Check sheet for the modelled part. Datum: model origin and axes. Units: mm. A direction names the side the tool comes from. Round coordinates to 2 decimals unless told otherwise and drop trailing zeros. Write each loop counter-clockwise with the first axis right and the second up, starting at its lowest first coordinate (ties: lowest second). Pieces come first, ordered by that corner, then holes.
Item 1: Cross-section at C-C on z = 0.65. Count the separate pieces of the cut face and the enclosed holes in it, plus the area to 3 significant figures.
Item 2: Release check for a two-part mould opening along Y. For faces 3 (the cylindrical face through (-38.72, 57.27, 0.99)), 4 (the cylindrical face through (41.02, 53.406, 1.014)), 5 (the cylindrical face through (31.9, 2.4, 1)) record: +Y half, -Y half, draft (parallel to the pull), parting line (faces both ways), or undercut.
Item 3: Cross-section at A-A on x = -12. Enter the section's corners in (y, z).
Item 4: Cross-section at B-B on y = 9. Enter the section's corners in (x, z), plus the area to 3 significant figures.
Item 5: Material ranges on line 1 (X direction, y = 46, z = 1.5); line 2 (X direction, y = 39.5, z = 1.3); line 3 (Y direction, x = 6.5, z = 1.3), recorded low to high.
Item 6: Cross-section at D-D on y = 65.5. Enter the section's corners in (x, z), plus the area to 3 significant figures.
Item 7: Tool access check on faces 1 (the flat face through (7.21, 73.23, 1.01)), 2 (the cylindrical face through (46.193, 31.142, 0.986)). Record the directions out of +Z, -Z, +X, -X, +Y, -Y that give a thin tool (end or side, any length) a straight path to the whole face; none if there is none.
Item 8: Go/stop test with flat-tipped pins: pin 1 Ø1 at (x, z) = (18.5, 0) entering from -Y; pin 2 Ø1 at (x, z) = (15, 1.5) entering from +Y. Record where each tip stops, or that it passes through.
Autodesk Inventor part; units mm, degrees
ref_plane "YZ Plane" through (0, 0, 0) normal (1, 0, 0) x (0, 1, 0)
ref_plane "XZ Plane" through (0, 0, 0) normal (0, 1, 0) x (-1, 0, 0)
ref_plane "XY Plane" through (0, 0, 0) normal (0, 0, 1) x (1, 0, 0)
ref_plane "Arbeitsebene1" through (0, 0, 0) normal (0, 0, 1) x (1, 0, 0)
sketch "Skizze1" plane through (0, 0, 0) normal (0, 0, 1) x (1, 0, 0)
  line L0 (39.3233, 58.7442) -> (31.1975, 48.5587)
  arc A0 (20.3661, 6.7006) -> (31.1975, 48.5587) centre (0, 34.301) ccw
  line L1 (20.3661, 6.7006) -> (24.3422, 1.3125)
  arc A1 (24.3422, 1.3125) -> (31.7994, 0.6471) centre (28.3654, 4.2814) ccw
  arc A2 (31.7994, 0.6471) -> (39.3233, 58.7442) centre (0, 34.301) ccw
  circle A3 centre (37.5836, 49.0481) radius 1.4
  circle A4 centre (39.9219, 28.2806) radius 1.4
  circle A5 centre (31.5631, 9.1262) radius 1.4
  line L2 (6.9617, 67.8882) -> (15.0883, 78.0746)
  arc A6 (15.0883, 78.0746) -> (-39.8826, 57.8205) centre (0, 34.301) ccw
  arc A7 (-39.8826, 57.8205) -> (-37.5755, 50.698) centre (-35.5757, 55.2807) ccw
  line L3 (-37.5755, 50.698) -> (-31.4381, 48.0198)
  arc A8 (6.9617, 67.8882) -> (-31.4381, 48.0198) centre (0, 34.301) ccw
  circle A9 centre (-31.5631, 59.4759) radius 1.4
  circle A10 centre (-14.7471, 71.8847) radius 1.4
  circle A11 centre (6.0205, 74.2229) radius 1.4
  circle A12 centre (-0.002, 34.3021) radius 3.35
  circle A13 centre (9.062, 45.6666) radius 3
  circle A14 centre (2.4174, 50.9675) radius 1.9
  circle A15 centre (15.7065, 40.3657) radius 1.9
  circle A16 centre (6.6446, 29.0001) radius 1.9
  circle A17 centre (-6.6446, 39.602) radius 1.9
  line L4 (31.7994, 0.6471) -> (-40.3324, 56.8214)
  arc A18 (20.3661, 6.7006) -> (-31.4381, 48.0198) centre (0, 34.301) ccw
  arc A19 (31.7994, 0.6471) -> (-39.8826, 57.8205) centre (0, 34.301) ccw
  circle A20 centre (15.7065, 40.3657) radius 1.4
  circle A21 centre (6.6446, 29.0001) radius 1.4
  circle A22 centre (-6.6446, 39.602) radius 1.4
  circle A23 centre (2.4174, 50.9675) radius 1.4
  point P0 (0, 0)
  dimension "d2" = 2.8
  dimension "d3" = 2.8
  dimension "d4" = 2.8
  dimension "d5" = 2.8
extrude "Extrusion1" add sketch "Skizze1" along normal blind 2 contours A2 L4 A0 L0 | L0 A18 L2 A19 | A0 L4 A8 A18 | L2 A8 L4 A7 A6 | A14 | A15 | A16 | A17
sketch "Skizze2" plane through (0, 0, 2) normal (0, 0, 1) x (1, 0, 0)
  arc A0 (31.7994, 0.6471) -> (-39.8826, 57.8205) centre (0, 34.301) ccw
  arc A1 (-39.8826, 57.8205) -> (-40.3324, 56.8214) centre (-35.5757, 55.2807) ccw
  line L0 (-40.3324, 56.8214) -> (31.7994, 0.6471)
  circle A2 centre (31.5631, 9.1262) radius 1.4
  circle A3 centre (39.9219, 28.2806) radius 1.4
  circle A4 centre (37.5836, 49.0481) radius 1.4
  circle A5 centre (-31.5631, 59.4759) radius 1.4
  circle A6 centre (-14.7471, 71.8847) radius 1.4
  circle A7 centre (6.0205, 74.2229) radius 1.4
  circle A8 centre (9.062, 45.6666) radius 3
  circle A9 centre (-0.002, 34.3021) radius 3.35
  circle A10 centre (15.7065, 40.3657) radius 1.4
  circle A11 centre (2.4174, 50.9675) radius 1.4
  circle A12 centre (-6.6446, 39.602) radius 1.4
  circle A13 centre (6.6446, 29.0001) radius 1.4
  line L1 (29.1054, 5.9703) -> (34.0209, 12.2821) construction
  circle A14 centre (31.5631, 9.1262) radius 1.4
  line L2 (30.3283, 5.018) -> (35.2438, 11.3297)
  line L3 (32.798, 13.2345) -> (27.8825, 6.9227)
  arc A15 (27.8825, 6.9227) -> (30.3283, 5.018) centre (29.1054, 5.9703) ccw
  arc A16 (35.2438, 11.3297) -> (32.798, 13.2345) centre (34.0209, 12.2821) ccw
  line L4 (37.4642, 25.1247) -> (42.3796, 31.4365) construction
  line L5 (38.6871, 24.1723) -> (43.6025, 30.4841)
  line L6 (41.1567, 32.3888) -> (36.2413, 26.0771)
  arc A17 (36.2413, 26.0771) -> (38.6871, 24.1723) centre (37.4642, 25.1247) ccw
  arc A18 (43.6025, 30.4841) -> (41.1567, 32.3888) centre (42.3796, 31.4365) ccw
  line L7 (35.1259, 45.8922) -> (40.0413, 52.204) construction
  line L8 (36.3488, 44.9399) -> (41.2642, 51.2516)
  line L9 (38.8184, 53.1564) -> (33.903, 46.8446)
  arc A19 (33.903, 46.8446) -> (36.3488, 44.9399) centre (35.1259, 45.8922) ccw
  arc A20 (41.2642, 51.2516) -> (38.8184, 53.1564) centre (40.0413, 52.204) ccw
  line L10 (3.5627, 71.0671) -> (8.4782, 77.3788) construction
  line L11 (4.7857, 70.1147) -> (9.7011, 76.4265)
  line L12 (7.2553, 78.3312) -> (2.3398, 72.0194)
  arc A21 (2.3398, 72.0194) -> (4.7857, 70.1147) centre (3.5627, 71.0671) ccw
  arc A22 (9.7011, 76.4265) -> (7.2553, 78.3312) centre (8.4782, 77.3788) ccw
  line L13 (-17.2048, 68.7288) -> (-12.2894, 75.0405) construction
  line L14 (-15.9819, 67.7764) -> (-11.0664, 74.0882)
  line L15 (-13.5123, 75.9929) -> (-18.4277, 69.6811)
  arc A23 (-18.4277, 69.6811) -> (-15.9819, 67.7764) centre (-17.2048, 68.7288) ccw
  arc A24 (-11.0664, 74.0882) -> (-13.5123, 75.9929) centre (-12.2894, 75.0405) ccw
  line L16 (-34.0209, 56.32) -> (-29.1054, 62.6318) construction
  line L17 (-32.798, 55.3676) -> (-27.8825, 61.6794)
  line L18 (-30.3283, 63.5841) -> (-35.2438, 57.2723)
  arc A25 (-35.2438, 57.2723) -> (-32.798, 55.3676) centre (-34.0209, 56.32) ccw
  arc A26 (-27.8825, 61.6794) -> (-30.3283, 63.5841) centre (-29.1054, 62.6318) ccw
  line L19 (29.1054, 5.9703) -> (34.0209, 12.2821) construction
  line L20 (30.3283, 5.018) -> (35.2438, 11.3297)
  line L21 (32.798, 13.2345) -> (27.8825, 6.9227)
  arc A27 (27.8825, 6.9227) -> (30.3283, 5.018) centre (29.1054, 5.9703) ccw
  arc A28 (35.2438, 11.3297) -> (32.798, 13.2345) centre (34.0209, 12.2821) ccw
  point P0 (0, 0)
  dimension "d6" = 4
  dimension "d7" = 3.1
  dimension "d8" = 3.1
  dimension "d9" = 3.1
  dimension "d10" = 3.1
  dimension "d11" = 3.1
  dimension "d12" = 3.1
  dimension "d13" = 3.1
extrude "Extrusion2" cut sketch "Skizze2" against normal blind 2 contours A7 | A15 L3 A16 L2 | A17 L6 A18 L5 | A19 L9 A20 L8 | A21 L12 A22 L11 | A23 L15 A24 L14 | A25 L18 A26 L17
fillet "Rundung1" radius 5 2 edges at (-40.3324, 56.8214, 1) (31.7994, 0.6471, 1)
properties part number "Anglerfish_Lightplate_Tosslink_adjuster_flipped"
Response values:
1. separate pieces: 1
1. enclosed holes: 12
1. area: 3,720 mm2
2. face 3: parting line
2. face 4: undercut
2. face 5: -Y half
3. outline: (34.76, 0) - (72.89, 0) - (72.89, 2) - (34.76, 2) - close; (76.56, 0) - (79.02, 0) - (79.02, 2) - (76.56, 2) - close
4. outline: (21.07, 0) - (29.5, 0) - (29.5, 2) - (21.07, 2) - close; (33.43, 0) - (38.78, 0) - (38.78, 2) - (33.43, 2) - close
4. area: 27.5 mm2
5. line 1: x = -26.44 to 6.08, 12.04 to 33.58, 37.17 to 44.8
5. line 2: x = -18.09 to -8.04, -5.25 to 14.61, 16.81 to 46.01
5. line 3: y = 20.35 to 27.61, 30.39 to 44.11, 47.23 to 72.32, 77.36 to 80.14
6. outline: (-34.21, 0) - (34.21, 0) - (34.21, 2) - (-34.21, 2) - close
6. area: 137 mm2
7. face 1: +Z, -Z
7. face 2: +Z, -Z, +X
8. pin 1: stops at y = 10.61
8. pin 2: stops at y = 78.27
